The drawing under review shows one solid part. Ordinate dimensions are in mm from its lowest x, y, z. Give positions to 0.01 mm unless a question says otherwise; leave off trailing zeros. Order: outer loops, then holes, each group sorted by start corner. A loop starts at its lowest first (then second) coordinate and runs counter-clockwise, first axis right, second up. Notation, with made-up numbers: (42.25, 13) -> (101.25, 13) arc R15 cw to (101.25, 23) -> close; hole circle Ø1 at (-9.75, 74). An arc over 180 degrees is marked (long way). One line per item, written item: value. Start each with the question number.
1) Wall thickness on line 1 along Y through (x, z) = (4.25, 1.8); line 2 along X through (y, z) = (4.5, 1.8); line 3 along X through (y, z) = (15.75, 0.9): over which ranges is each line inside the solid? List them lowest first. Write a range as from..to.
2) Consider section B-B (x = 5). State the section outline as (y, z) points.
3) Consider section C-C (z = 1.15). State the section outline as (x, y) points.
4) Consider section D-D (y = 5.5). State the section outline as (x, z) points, plus the area to 3 significant figures.
5) The part is to be moulded in two halves that separate along X. For the marked faces 1, 2, 3 and 4, say which applies: released by +X, released by -X, zero draft, split by the parting line, or undercut.
6) Consider section A-A (y = 15). State the section outline as (x, z) points, plus the area to 3 significant figures.
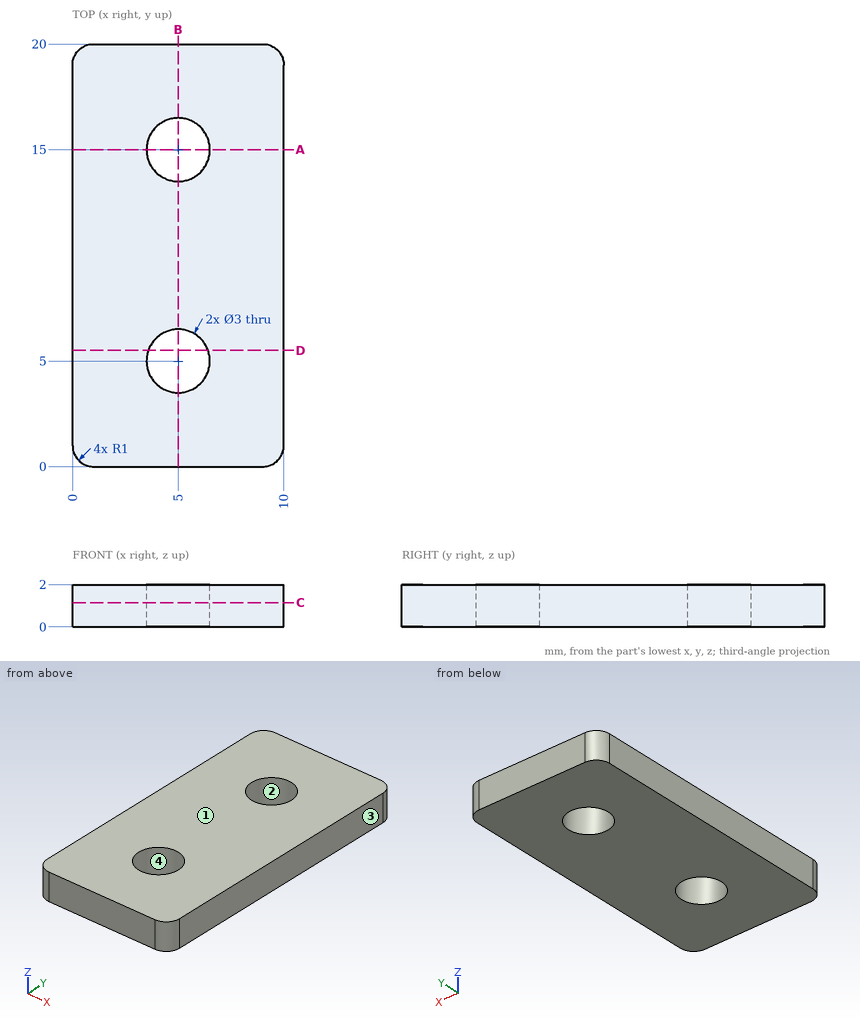
Checked values:
1. line 1: y = 0..3.7, 6.3..13.7, 16.3..20
1. line 2: x = 0..3.59, 6.41..10
1. line 3: x = 0..3.7, 6.3..10
2. outline: (0, 0) -> (3.5, 0) -> (3.5, 2) -> (0, 2) -> close; (6.5, 0) -> (13.5, 0) -> (13.5, 2) -> (6.5, 2) -> close; (16.5, 0) -> (20, 0) -> (20, 2) -> (16.5, 2) -> close
3. outline: (0, 1) arc R1 ccw to (1, 0) -> (9, 0) arc R1 ccw to (10, 1) -> (10, 19) arc R1 ccw to (9, 20) -> (1, 20) arc R1 ccw to (0, 19) -> close; hole circle Ø3 at (5, 5); hole circle Ø3 at (5, 15)
4. outline: (0, 0) -> (3.59, 0) -> (3.59, 2) -> (0, 2) -> close; (6.41, 0) -> (10, 0) -> (10, 2) -> (6.41, 2) -> close
4. area: 14.3 mm^2
5. face 1: zero draft
5. face 2: undercut
5. face 3: released by +X
5. face 4: undercut
6. outline: (0, 0) -> (3.5, 0) -> (3.5, 2) -> (0, 2) -> close; (6.5, 0) -> (10, 0) -> (10, 2) -> (6.5, 2) -> close
6. area: 14.0 mm^2
